Can you work these out from the drawing? Everything is in mm from the part's minimum corner. Round coordinates to 2 decimals unless told otherwise and drop trailing zeros. Write each loop counter-clockwise with the first axis right and the second up, starting at its lowest first coordinate (ties: lowest second). Pieces come first, ordered by that corner, then holes.
Q1. I'm going to push flat-ended pins straight in: pin 1 Ø2 at (x, y) = (103.5, 25.5) entering from -Z; pin 2 Ø1.5 at (y, z) = (120.5, 5) entering from +X (1 decimal); pin 3 Ø4 at (x, z) = (84, 8.5) entering from +Y; pin 4 Ø2 at (y, z) = (55, 1.5) entering from -X. Where does each tip first touch, or does it pass through?
Q2. If we section it at C-C (z = 5): Please give me the cut outline in (x, y), plus the area to 3 significant figures.
Q3. If we section it at D-D (y = 70): Please give me the cut outline in (x, z), plus the area to 3 significant figures.
Q4. If we section it at B-B (y = 130): Please give me the cut outline in (x, z) (1 decimal).
Q5. Please list where these lines run through material, in increasing order: line 1 along Y through (x, z) = (70, 1.4); line 2 along X through (y, z) = (69, 0.5); line 3 along Z through (x, y) = (76, 24).
Q6. We'd pull the mould along Y, two halves only. Please class the marked faces 1 and 2: +Y half, -Y half, draft (parallel to the pull), parting line (faces both ways), or undercut.
Q7. If we section it at A-A (x = 70): Please give me the cut outline in (y, z), plus the area to 3 significant figures.
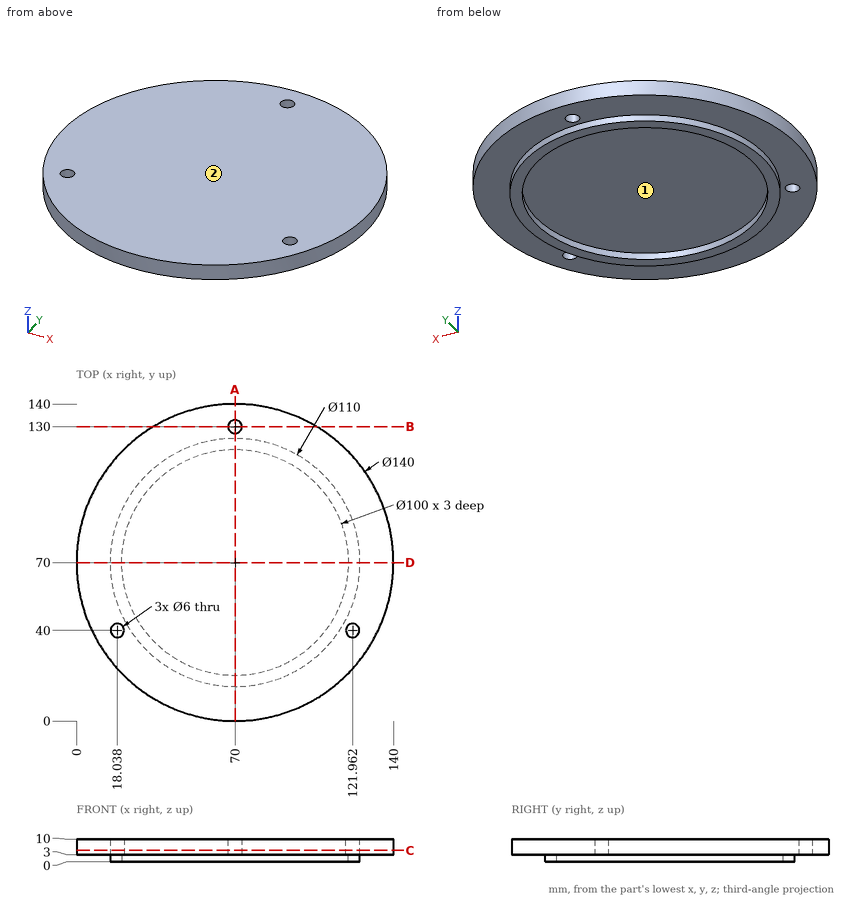
A:
1. pin 1: stops at z = 0
1. pin 2: stops at x = 119.2
1. pin 3: stops at y = 138.96
1. pin 4: stops at x = 16.81
2. outline: circle Ø140 at (70, 70); hole circle Ø6 at (18.04, 40); hole circle Ø6 at (70, 130); hole circle Ø6 at (121.96, 40)
2. area: 15,300 mm2
3. outline: (0, 3) - (15, 3) - (15, 0) - (20, 0) - (20, 3) - (120, 3) - (120, 0) - (125, 0) - (125, 3) - (140, 3) - (140, 10) - (0, 10) - close
3. area: 1,010 mm2
4. outline: (33.9, 3) - (67, 3) - (67, 10) - (33.9, 10) - close; (73, 3) - (106.1, 3) - (106.1, 10) - (73, 10) - close
5. line 1: y = 15 to 20, 120 to 125
5. line 2: x = 15.01 to 20.01, 119.99 to 124.99
5. line 3: z = 3 to 10
6. face 1: undercut
6. face 2: draft
7. outline: (0, 3) - (15, 3) - (15, 0) - (20, 0) - (20, 3) - (120, 3) - (120, 0) - (125, 0) - (125, 3) - (127, 3) - (127, 10) - (0, 10) - close; (133, 3) - (140, 3) - (140, 10) - (133, 10) - close
7. area: 968 mm2
